```python
from build123d import *

# Parameters (mm, degrees)
F2_SIZE   = 0.7
F3_SIZE   = 0.2
F4_W      = 1
F4_H      = 14
F6_DEPTH  = 7.5
F7_W      = 1.2
F7_H      = 14
F8_DEPTH  = 7.5
F9_W      = 0.8
F9_H      = 14
F10_DEPTH = 7.5


# Not quite as in the source:
# - a fillet or chamfer that OpenCascade refuses, or shapes differently, is made with other operations: its cross-section is extruded or revolved along the edge and cut away or added


with BuildPart() as f1:
    # F0 (on Front) → F1 (revolve)
    with BuildSketch(Plane.XZ):
        Polygon((0, 7.5), (0, 0), (40, 0), (40, 7.5), (11, 7.5), (11, 6), (5, 6), (5, 7.5), align=None)
    revolve(axis=Axis((20, 0, 0), (1, 0, 0)))

    # F2
    f2_edges = [f1.edges().sort_by_distance(p)[0] for p in [
        (0, 0, -7.5),
    ]]
    chamfer(f2_edges, length=F2_SIZE)

    # F3
    f3_edges = [f1.edges().sort_by_distance(p)[0] for p in [
        (5, 0, -7.5),
        (11, 0, -7.5),
    ]]
    chamfer(f3_edges, length=F3_SIZE)

    # F5: chamfer of 0.4 on 3 edges, made by hand

    # F5_s1 → F5_t2 (revolve, cut)
    with BuildSketch(Plane.XZ):
        Polygon((11.0828427125, 7.3828427125), (11.3656854249, 7.5), (11.2, 7.5), align=None)
    revolve(axis=Axis((11.2, 0, 0), (1, 0, 0)), mode=Mode.SUBTRACT)

    # F5_s3 → F5_t4 (revolve, cut)
    with BuildSketch(Plane.XZ):
        Polygon((39.6, 7.5), (40, 7.1), (40, 7.5), align=None)
    revolve(axis=Axis((40, 0, 0), (1, 0, 0)), mode=Mode.SUBTRACT)

    # F4 (on Front) → F6 (cut)
    with BuildSketch(Plane.XZ):
        with Locations((35.5, 0)):
            Rectangle(F4_W, F4_H)
    extrude(amount=F6_DEPTH, mode=Mode.SUBTRACT)

    # F7 (on Top) → F8 (cut)
    with BuildSketch(Plane.XY):
        with Locations((32.8, 0)):
            Rectangle(F7_W, F7_H)
    extrude(amount=F8_DEPTH, mode=Mode.SUBTRACT)

    # F9 (on Top) → F10 (cut)
    with BuildSketch(Plane.XY):
        with Locations((37.6, 0)):
            Rectangle(F9_W, F9_H)
    extrude(amount=-F10_DEPTH, mode=Mode.SUBTRACT)


solid = f1.part
```
Read the model definition and answer for the solid it produces. Units are mm, in the model's axes. A direction names the side the tool comes from. Give positions to 0.01 mm unless a question says otherwise; leave off trailing zeros. Loops run counter-clockwise (first coordinate to the right, second up) from the corner with the lowest first, then second, coordinate; pieces in that order, holes last.
Item 1: For faces 1 (the flat face through (38, 0, -3)), 2 (the flat face through (35.5, 0, 0.1)), 3 (the flat face through (33, -7, 1)), determine the directions among +Z, -Z, +X, -X, +Y, -Y from which every point of the face is accessible in a straight line to the end or side of a thin tool.
Item 2: Each of these flat-tipped pins is pushed along its axis until it touches: pin 1 Ø1 at (x, z) = (32.5, 1.5) entering from -Y; pin 2 Ø5 at (x, z) = (23, 0.5) entering from -Y; pin 3 Ø0.6 at (x, z) = (32.5, 1.5) entering from +Y; pin 4 Ø4 at (x, y) = (8.5, -6) entering from -Z. Where does it stop, or does it pass through?
Item 3: Find the intervals of material crossed by line 1 along X through (y, z) = (3.5, -5.25); line 2 along X through (y, z) = (-0.5, -6.75); line 3 along X through (y, z) = (-1, 2.75), in increasing order.
Item 4: The mould has two halves that part along Z. Classify faces 4 (the flat face through (0, 0, 0)), 5 (the flat face through (36, -3, 0)), 6 (the flat face through (33, 0, 0)): released by +Z, released by -Z, zero draft, split by the parting line, or undercut.
Item 5: The part is cut by section A-A (x = 17). Write down the section's boundary in (y, z).
Taken from the geometry:
1. face 1: -Z
1. face 2: -Y
1. face 3: +Z
2. pin 1: stops at y = -7.43
2. pin 2: stops at y = -7.5
2. pin 3: stops at y = 7.4
2. pin 4: stops at z = -4.47
3. line 1: x = 0 to 5, 11 to 37.2, 38 to 40
3. line 2: x = 0 to 5, 11 to 35, 36 to 37.2, 38 to 40
3. line 3: x = 0 to 32.2, 33.4 to 35, 36 to 40
4. face 4: zero draft
4. face 5: undercut
4. face 6: released by +Z
5. outline: circle Ø15 at (0, 0)
